from build123d import *

# Parameters (mm, degrees)
SKETCH2_R                = 19.05
BOSS_EXTRUDE1_DEPTH      = 0.889
BOSS_EXTRUDE1_DEPTH_BACK = 0.889
SKETCH4_R                = 4.7625
CUT_EXTRUDE1_DEPTH       = 2.778
SKETCH5_R                = 0.79375
CUT_EXTRUDE2_DEPTH       = 2.778


with BuildPart() as part:
    # Sketch2 → Boss-Extrude1 (new body, two sides)
    with BuildSketch(Plane(origin=(0, 0, 0), x_dir=(1, 0, 0), z_dir=(0, 1, 0))) as boss_extrude1_sk:
        Circle(SKETCH2_R)
    extrude(amount=BOSS_EXTRUDE1_DEPTH)
    extrude(boss_extrude1_sk.sketch, amount=-BOSS_EXTRUDE1_DEPTH_BACK)

    # Sketch4 → Cut-Extrude1 (cut, through all)
    with BuildSketch(Plane(origin=(0, 0.889, 0), x_dir=(1, 0, 0), z_dir=(0, 1, 0))):
        Circle(SKETCH4_R)
    extrude(amount=-CUT_EXTRUDE1_DEPTH, mode=Mode.SUBTRACT)

    # Sketch5 → Cut-Extrude2 (cut, through all)
    with BuildSketch(Plane.XZ.offset(0.889)):
        with Locations((0, 6.604)):
            Circle(SKETCH5_R)
        with Locations((5.719231767, -3.302)):
            Circle(SKETCH5_R)
        with Locations((-5.719231767, -3.302)):
            Circle(SKETCH5_R)
    extrude(amount=-CUT_EXTRUDE2_DEPTH, mode=Mode.SUBTRACT)


solid = part.part
Model file for the job. Use its own axes, mm. Coordinates: 2 decimals unless noted, no trailing zeros. Write each loop counter-clockwise with the first axis right and the second up, starting at its lowest first coordinate (ties: lowest second). Pieces come first, ordered by that corner, then holes. Notation, with made-up numbers: (-30, 55) - (16, 55) arc R22 ccw to (16, 73) - close; hole circle Ø9 at (-28, 8). An arc over 180 degrees is marked (long way). Write each question's results on one line, items separated by ' | '. Start each with the question number.
1) Flat gauge pins, fed straight in: P1, Ø1, axis at y = 0.5, z = -14, coming from the +X side; P2, Ø1, axis at y = -0.5, z = 8.5, coming from the +X side. Where does each tip first touch, or does it go through?
2) Cut at A-A (z = 0). Write the cut outline in (x, y), then the cut area to 3 significant figures.
3) Probe line 1 along Z through (x, y) = (0, -0.1); line 2 along X through (y, z) = (0.15, -3); line 3 along Z through (x, y) = (1, -0.55). List the from-to ranges inside material, lowest first. Write a range as from..to.
4) Cut at B-B (x = 0). Write the cut outline in (y, z), then the cut area to 3 significant figures.
5) Mould opens along Z. For faces 1 (the face through (-3.78, 0.01, 2.9)), 2 (the face through (-15.12, 0.01, 11.59)), 3 (the face through (4, -0.889, 4)) say: pulls with the +Z half, pulls with the -Z half, needs draft (parallel to the pull), parting line crosses it, or undercut.
6) Cut at C-C (y = -0.35). Count the separate pieces of the cut face and the enclosed holes in it, then the cut area to 3 significant figures.
7) Cut at D-D (x = 13). Write the cut outline in (y, z), then the cut area to 3 significant figures.
Returned:
1) P1: x = 13.44 | P2: x = 17.29
2) outline: (-19.05, -0.89) - (-4.76, -0.89) - (-4.76, 0.89) - (-19.05, 0.89) - close; (4.76, -0.89) - (19.05, -0.89) - (19.05, 0.89) - (4.76, 0.89) - close | area: 50.8 mm^2
3) line 1: -19.05..-4.76, 4.76..5.81, 7.4..19.05 | line 2: -18.81..-6.45, -4.99..-3.7, 3.7..4.99, 6.45..18.81 | line 3: -19.02..-4.66, 4.66..19.02
4) outline: (-0.89, -19.05) - (0.89, -19.05) - (0.89, -4.76) - (-0.89, -4.76) - close; (-0.89, 4.76) - (0.89, 4.76) - (0.89, 5.81) - (-0.89, 5.81) - close; (-0.89, 7.4) - (0.89, 7.4) - (0.89, 19.05) - (-0.89, 19.05) - close | area: 48.0 mm^2
5) face 1: undercut | face 2: parting line crosses it | face 3: needs draft
6) separate pieces: 1 | enclosed holes: 4 | area: 1,060 mm^2
7) outline: (-0.89, -13.92) - (0.89, -13.92) - (0.89, 13.92) - (-0.89, 13.92) - close | area: 49.5 mm^2
